```python
from build123d import *

# Parameters (mm, degrees)
F0_R     = 11.2
F1_DEPTH = 7


with BuildPart() as f1:
    # F0 (on Top) → F1 (new body)
    with BuildSketch(Plane.XY):
        with BuildLine():
            ThreePointArc((1.625641, 13.099515), (9.331043, 9.336575), (13.098549, 1.633405))
            ThreePointArc((13.098549, 1.633405), (14.54896, 6.209741), (17.540058, 9.964721))
            ThreePointArc((17.540058, 9.964721), (13.833044, 13.839076), (10.039052, 17.628298))
            ThreePointArc((10.039052, 17.628298), (6.256496, 14.575938), (1.625641, 13.099515))
        make_face()
        with BuildLine():
            ThreePointArc((13.098549, 1.633405), (13.174613, 0.818276), (13.2, 0))
            ThreePointArc((13.2, 0), (13.174613, -0.818276), (13.098549, -1.633405))
            ThreePointArc((13.098549, -1.633405), (14.548449, -6.208782), (17.538418, -9.963296))
            ThreePointArc((17.538418, -9.963296), (31.671832, -12.011132), (39.397098, 0))
            ThreePointArc((39.397098, 0), (31.672821, 12.010681), (17.540058, 9.964721))
            ThreePointArc((17.540058, 9.964721), (14.54896, 6.209741), (13.098549, 1.633405))
        make_face()
        with Locations((26.197098, 0)):
            Circle(F0_R, mode=Mode.SUBTRACT)
        with BuildLine():
            ThreePointArc((-1.625641, 13.099515), (0, 13.2), (1.625641, 13.099515))
            ThreePointArc((1.625641, 13.099515), (6.256496, 14.575938), (10.039052, 17.628298))
            ThreePointArc((10.039052, 17.628298), (12.384577, 21.631508), (13.2, 26.19903))
            ThreePointArc((13.2, 26.19903), (-3.51391, 38.922726), (-11.329158, 19.4248))
            ThreePointArc((-11.329158, 19.4248), (-7.20826, 15.140956), (-1.625641, 13.099515))
        make_face()
        with Locations((0, 26.19903)):
            Circle(F0_R, mode=Mode.SUBTRACT)
        with BuildLine():
            ThreePointArc((-13.103194, 1.595718), (-9.344462, 9.323144), (-1.625641, 13.099515))
            ThreePointArc((-1.625641, 13.099515), (-7.20826, 15.140956), (-11.329158, 19.4248))
            ThreePointArc((-11.329158, 19.4248), (-14.678509, 14.841206), (-18.770392, 10.906235))
            ThreePointArc((-18.770392, 10.906235), (-14.930927, 6.863235), (-13.103194, 1.595718))
        make_face()
        with BuildLine():
            ThreePointArc((-13.103194, -1.595718), (-13.2, 0), (-13.103194, 1.595718))
            ThreePointArc((-13.103194, 1.595718), (-14.930927, 6.863235), (-18.770392, 10.906235))
            ThreePointArc((-18.770392, 10.906235), (-39.406354, 0.029513), (-18.819234, -10.939377))
            ThreePointArc((-18.819234, -10.939377), (-14.9463, -6.888428), (-13.103194, -1.595718))
        make_face()
        with Locations((-26.206387, 0)):
            Circle(F0_R, mode=Mode.SUBTRACT)
        with BuildLine():
            ThreePointArc((13.098549, -1.633405), (12.997098, 0), (13.098549, 1.633405))
            ThreePointArc((13.098549, 1.633405), (9.331043, 9.336575), (1.625641, 13.099515))
            ThreePointArc((1.625641, 13.099515), (0, 12.99903), (-1.625641, 13.099515))
            ThreePointArc((-1.625641, 13.099515), (-9.344462, 9.323144), (-13.103194, 1.595718))
            ThreePointArc((-13.103194, 1.595718), (-13.030611, 0.799326), (-13.006387, 0))
            ThreePointArc((-13.006387, 0), (-13.030611, -0.799326), (-13.103194, -1.595718))
            ThreePointArc((-13.103194, -1.595718), (-9.403382, -9.263714), (-1.791606, -13.07785))
            ThreePointArc((-1.791606, -13.07785), (0, -12.955699), (1.791606, -13.07785))
            ThreePointArc((1.791606, -13.07785), (9.390048, -9.27723), (13.098549, -1.633405))
        make_face()
        Circle(F0_R, mode=Mode.SUBTRACT)
        with BuildLine():
            ThreePointArc((-11.598392, -19.853533), (-7.503365, -15.295703), (-1.791606, -13.07785))
            ThreePointArc((-1.791606, -13.07785), (-9.403382, -9.263714), (-13.103194, -1.595718))
            ThreePointArc((-13.103194, -1.595718), (-14.9463, -6.888428), (-18.819234, -10.939377))
            ThreePointArc((-18.819234, -10.939377), (-14.994912, -15.223186), (-11.598392, -19.853533))
        make_face()
        with BuildLine():
            ThreePointArc((11.598392, -19.853533), (7.503365, -15.295703), (1.791606, -13.07785))
            ThreePointArc((1.791606, -13.07785), (0, -13.2), (-1.791606, -13.07785))
            ThreePointArc((-1.791606, -13.07785), (-7.503365, -15.295703), (-11.598392, -19.853533))
            ThreePointArc((-11.598392, -19.853533), (-3.251248, -38.949033), (13.2, -26.155699))
            ThreePointArc((13.2, -26.155699), (12.793334, -22.904451), (11.598392, -19.853533))
        make_face()
        with Locations((0, -26.155699)):
            Circle(F0_R, mode=Mode.SUBTRACT)
        with BuildLine():
            ThreePointArc((17.538418, -9.963296), (14.548449, -6.208782), (13.098549, -1.633405))
            ThreePointArc((13.098549, -1.633405), (9.390048, -9.27723), (1.791606, -13.07785))
            ThreePointArc((1.791606, -13.07785), (7.503365, -15.295703), (11.598392, -19.853533))
            ThreePointArc((11.598392, -19.853533), (14.246289, -14.714953), (17.538418, -9.963296))
        make_face()
    extrude(amount=F1_DEPTH)


solid = f1.part
```
Source: CAD feature listing. Evaluate the final solid. Frame: model axes, mm. A direction names the side the tool comes from. Coordinates: 2 decimals unless noted, no trailing zeros. Loops run counter-clockwise (first coordinate to the right, second up) from the corner with the lowest first, then second, coordinate; pieces in that order, holes last. Notation, with made-up numbers: M 28,32 L 72,32 A16 cw 72,44 Z; hole C -32,35.5 d9. An arc over 180 degrees is marked long. Put each result on its own line as item: value. Start each with the question number.
1) Cut plane B-B on z = 4.5. Give the number of separate pieces and of enclosed holes in the cut face, then the cut area to 3 significant figures.
2) Pull-direction query (Z, two-part tool) for faces 3 (the face through (-0.2, -11.5, 0)), 4 (the face through (-15.046, -15.161, 3.451)), 5 (the face through (-0.2, -11.5, 7)); classes: pulls with the +Z half, pulls with the -Z half, needs draft (parallel to the pull), parting line crosses it, or undercut.
3) Cut plane C-C on x = 29. Return the cut outline in (y, z).
4) Cut plane D-D on y = 4.5. Return the cut outline in (x, z), then the cut area to 3 significant figures.
5) Ray query, L1, parallel to X at y = 11.5, z = 4; L2, parallel to Y at x = -7, z = 2.25; L3, parallel to Y at x = 20, z = 6. Return the intervals inside material, ascending. Write a range as from..to.
6) Contact query for flat-ended pins moving along their axis: pin 1 Ø4 at (x, z) = (10, 3) entering from +Y; pin 2 Ø13.5 at (x, y) = (-26.21, 0) entering from +Z; pin 3 Ø1.5 at (y, z) = (-28.5, 3.5) entering from -X; pin 4 Ø4 at (x, z) = (23, 1) entering from +Y. Output: stop coordinate, or through.
7) Reachability of faces 1 (the face through (12.805, -22.949, 3.451)), 2 (the face through (-14.626, 14.901, 3.451)) from +Z, -Z, +X, -X, +Y, -Y: full face, straight path, thin tool, end or side. Return the list, or none.
8) Cut plane A-A on x = 0. Return the cut outline in (y, z).
The answers:
1. separate pieces: 1
1. enclosed holes: 9
1. area: 1,130 mm²
2. face 3: pulls with the -Z half
2. face 4: needs draft
2. face 5: pulls with the +Z half
3. outline: M -12.9,0 L -10.84,0 L -10.84,7 L -12.9,7 Z; M 10.84,0 L 12.9,0 L 12.9,7 L 10.84,7 Z
4. outline: M -38.62,0 L -36.46,0 L -36.46,7 L -38.62,7 Z; M -15.95,0 L -10.26,0 L -10.26,7 L -15.95,7 Z; M 10.26,0 L 15.94,0 L 15.94,7 L 10.26,7 Z; M 36.45,0 L 38.61,0 L 38.61,7 L 36.45,7 Z
4. area: 110 mm²
5. L1: x = -32.69..-19.73, -18.06..16.09, 19.72..32.68
5. L2: y = -37.35..-34.9, -17.41..-8.74, 8.74..17.46, 34.94..37.39
5. L3: y = -11.65..-9.33, 9.33..11.65
6. pin 1: stops at y = 36.7
6. pin 2: passes through
6. pin 3: stops at x = -13.1
6. pin 4: stops at y = 13.15
7. face 1: +Z, -Z, +X
7. face 2: +Z, -Z
8. outline: M -39.36,0 L -37.36,0 L -37.36,7 L -39.36,7 Z; M -14.96,0 L -13.2,0 L -13.2,7 L -14.96,7 Z; M -12.96,0 L -11.2,0 L -11.2,7 L -12.96,7 Z; M 11.2,0 L 13,0 L 13,7 L 11.2,7 Z; M 13.2,0 L 15,0 L 15,7 L 13.2,7 Z; M 37.4,0 L 39.4,0 L 39.4,7 L 37.4,7 Z
